Could you check a few things on this model? Use its own coordinates, in mm. Face numbers are marked on the shaded views. Give positions to 0.01 mm unless a question says otherwise; leave off trailing zeros. Order: outer loops, then holes, each group sorted by start corner. A loop starts at its lowest first (then second) coordinate and runs counter-clockwise, first axis right, second up.
(1) Imagine slicing it at C-C, the plane z = 10. Write out the boundary of the cut face in (x, y).
(2) Imagine slicing it at A-A, the plane y = 0. Write out the boundary of the cut face in (x, z).
(3) Imagine slicing it at D-D, the plane z = 45. Write out the boundary of the cut face in (x, y).
(4) If we mould it in two halves opening along Y, with no side actions, what happens to the marked faces 1, 2 and 3? For each: released by +Y, released by -Y, zero draft, split by the parting line, or undercut.
(5) If I drill on probe 1 along Y at (x, z) = (0, 24); probe 2 along X at (y, z) = (10, 3.5); probe 3 along Y at (x, z) = (0, 37) (3 decimals), over which ranges is the centre line in solid material (lowest first)?
(6) Will these pins go through, and if not, where does the flat tip stop? pin 1 (8 mm diameter, centred on x = 52, y = -32.5, fed in from -Z); pin 2 (10 mm diameter, centred on y = 18, z = 16, fed in from +X); pin 3 (1.5 mm diameter, centred on x = -8, z = 5.5, fed in from -Y).
from build123d import *

# Parameters (mm, degrees)
SKETCH1_R           = 75
BOSS_EXTRUDE1_DEPTH = 50
FILLET2_R           = 20
FILLET3_R           = 20
SKETCH2_R           = 12.5
CUT_EXTRUDE1_DEPTH  = 51


with BuildPart() as part:
    # Sketch1 → Boss-Extrude1 (new body)
    with BuildSketch(Plane.XY):
        Circle(SKETCH1_R)
    extrude(amount=BOSS_EXTRUDE1_DEPTH)

    # Fillet2
    fillet2_edges = [part.edges().sort_by_distance(p)[0] for p in [
        (-75, 0, 50),
    ]]
    fillet(fillet2_edges, radius=FILLET2_R)

    # Fillet3
    fillet3_edges = [part.edges().sort_by_distance(p)[0] for p in [
        (-75, 0, 0),
    ]]
    fillet(fillet3_edges, radius=FILLET3_R)

    # Sketch2 → Cut-Extrude1 (cut, through all)
    with BuildSketch(Plane.XY.offset(50)):
        Circle(SKETCH2_R)
    extrude(amount=-CUT_EXTRUDE1_DEPTH, mode=Mode.SUBTRACT)


solid = part.part
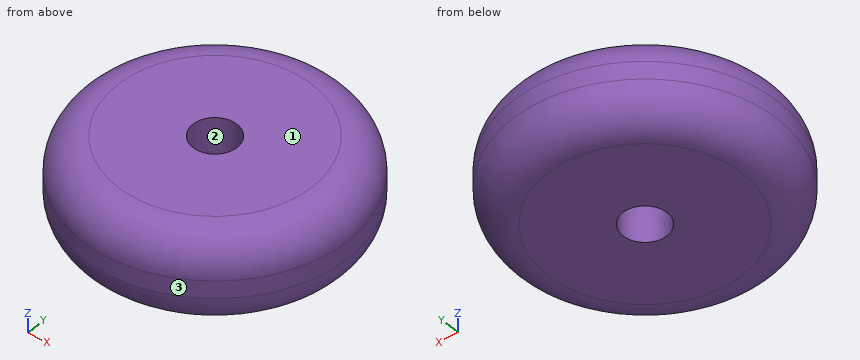
Answer block:
1. outline: circle Ø144.64 at (0, 0); hole circle Ø25 at (0, 0)
2. outline: (-75, 20) arc R20 ccw to (-55, 0) - (-12.5, 0) - (-12.5, 50) - (-55, 50) arc R20 ccw to (-75, 30) - close; (12.5, 0) - (55, 0) arc R20 ccw to (75, 20) - (75, 30) arc R20 ccw to (55, 50) - (12.5, 50) - close
3. outline: circle Ø136.46 at (0, 0); hole circle Ø25 at (0, 0)
4. face 1: zero draft
4. face 2: undercut
4. face 3: split by the parting line
5. probe 1: y = -75 to -12.5, 12.5 to 75
5. probe 2: x = -65.54 to -7.5, 7.5 to 65.54
5. probe 3: y = -73.735 to -12.5, 12.5 to 73.735
6. pin 1: stops at z = 0.14
6. pin 2: stops at x = 73.69
6. pin 3: stops at y = -69.07
